Geometry check sheet. Reference: drawing and pictorial views, mm from the part's lowest x, y, z. A direction names the side the tool comes from. Round coordinates to 2 decimals unless told otherwise and drop trailing zeros. Write each loop counter-clockwise with the first axis right and the second up, starting at its lowest first coordinate (ties: lowest second). Pieces come first, ordered by that corner, then holes. Notation, with made-up numbers: M -12,77.5 L 6,77.5 A5 ccw 6,83.5 Z; hole C 58,-27.75 d5. An arc over 180 degrees is marked long. Put each result on its own line as item: value. Start each with the question number.
(1) Tool access check on the marked faces 5, 6 and 7. Record the directions out of +Z, -Z, +X, -X, +Y, -Y that give a thin tool (end or side, any length) a straight path to the whole face; none if there is none.
(2) Section check C-C on z = 7.75. Record the cut outline in (x, y).
(3) Mould release check, pull along Z, two halves, no side actions. Record for the marked faces 1, 2, 3 and 4: pulls with the +Z half, pulls with the -Z half, needs draft (parallel to the pull), parting line crosses it, or undercut.
(4) Section check A-A on z = 4.5. Record the cut outline in (x, y).
(5) Section check B-B on x = 1.5. Record the cut outline in (y, z), then the cut area to 3 significant figures.
(6) Gauge pin test, flat end, axial feed: pin 1 (3 mm diameter, centred on x = 8, z = 3.5, fed in from +Y). Record the tip position at first contact, or that the pin passes through.
(7) Material ranges on probe 1 along Z at (x, y) = (0.5, 54.5); probe 2 along X at (y, z) = (36.5, 7.25); probe 3 along Y at (x, z) = (1.5, 4), recorded low to high.
(8) Section check D-D on y = 38. Record the cut outline in (x, z), then the cut area to 3 significant figures.
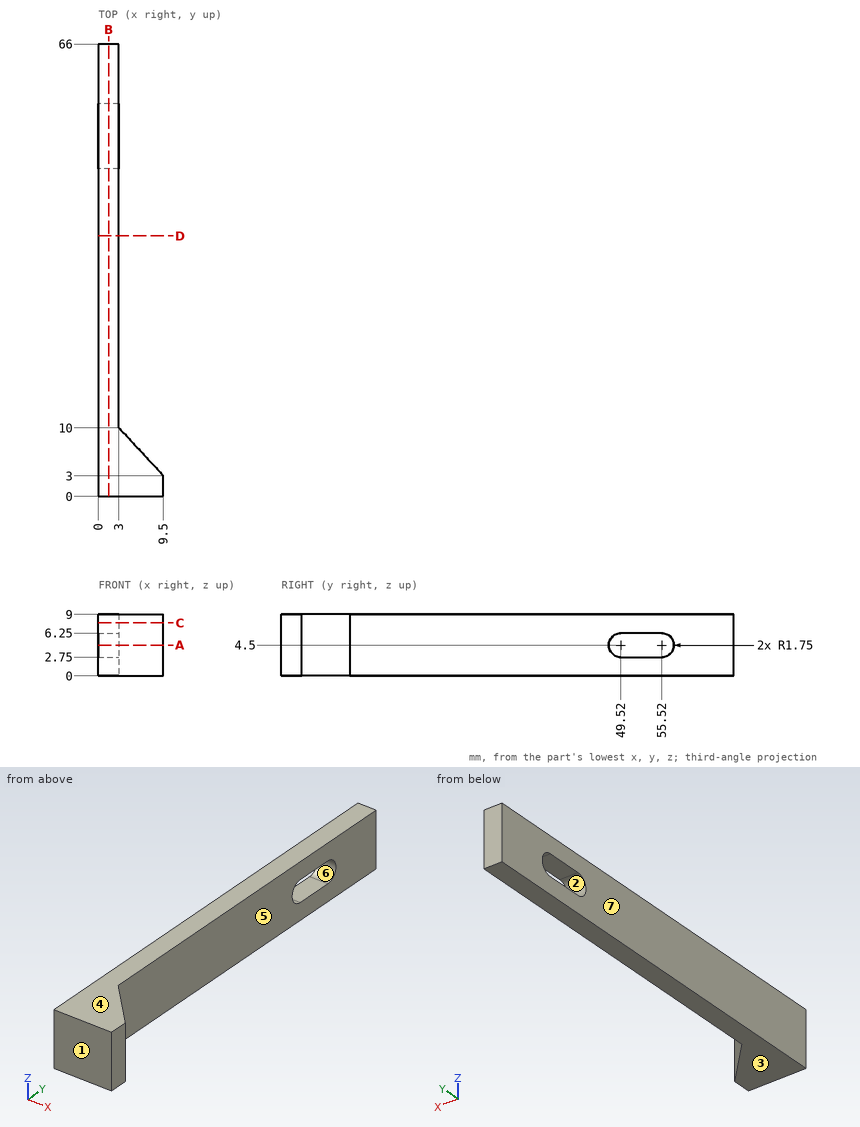
Answers follow:
1. face 5: +Z, -Z, +X, +Y
1. face 6: +X, -X
1. face 7: +Z, -Z, -X, +Y, -Y
2. outline: M 0,0 L 9.5,0 L 9.5,3 L 3,10 L 3,66 L 0,66 Z
3. face 1: needs draft
3. face 2: undercut
3. face 3: pulls with the -Z half
3. face 4: pulls with the +Z half
4. outline: M 0,0 L 9.5,0 L 9.5,3 L 3,10 L 3,47.77 L 0,47.77 Z; M 0,57.27 L 3,57.27 L 3,66 L 0,66 Z
5. outline: M 0,0 L 66,0 L 66,9 L 0,9 Z; hole M 49.52,2.75 L 55.52,2.75 A1.75 ccw 55.52,6.25 L 49.52,6.25 A1.75 ccw Z
5. area: 563 mm^2
6. pin 1: stops at y = 6.23
7. probe 1: z = 0 to 2.75, 6.25 to 9
7. probe 2: x = 0 to 3
7. probe 3: y = 0 to 47.84, 57.2 to 66
8. outline: M 0,0 L 3,0 L 3,9 L 0,9 Z
8. area: 27.0 mm^2
